```python
from build123d import *

# Parameters (mm, degrees)
SKETCH1_W           = 230
SKETCH1_H           = 25
BOSS_EXTRUDE1_DEPTH = 150
SKETCH2_W           = 210
SKETCH2_H           = 130
CUT_EXTRUDE1_DEPTH  = 20
SKETCH4_W           = 6.527967864
SKETCH4_H           = 110
BOSS_EXTRUDE3_DEPTH = 30
CUT_EXTRUDE2_REACH  = 7
SKETCH5_R           = 1.35
SKETCH5_R_2         = 1.5
SKETCH6_R           = 1.5
CUT_EXTRUDE3_DEPTH  = 6
CUT_EXTRUDE4_REACH  = 232
SKETCH7_R           = 3.25
CUT_EXTRUDE5_REACH  = 12
SKETCH8_R           = 3.25
SKETCH9_W           = 4.75
SKETCH9_H           = 80
BOSS_EXTRUDE4_DEPTH = 10
SKETCH10_R          = 2
CUT_EXTRUDE6_DEPTH  = 10
SKETCH11_R          = 2
CUT_EXTRUDE7_DEPTH  = 10
SKETCH12_W          = 3.25
SKETCH12_H          = 7.5
CUT_EXTRUDE8_DEPTH  = 8.5
SKETCH13_W          = 4.75
SKETCH13_H          = 1
CUT_EXTRUDE9_DEPTH  = 10


with BuildPart() as part:
    # Sketch1 → Boss-Extrude1 (new body)
    with BuildSketch(Plane.XY):
        with Locations((115, 12.5)):
            Rectangle(SKETCH1_W, SKETCH1_H)
    extrude(amount=BOSS_EXTRUDE1_DEPTH)

    # Sketch2 → Cut-Extrude1 (cut)
    with BuildSketch(Plane(origin=(0, 25, 0), x_dir=(1, 0, 0), z_dir=(0, 1, 0))):
        with Locations((115, -75)):
            Rectangle(SKETCH2_W, SKETCH2_H)
    extrude(amount=-CUT_EXTRUDE1_DEPTH, mode=Mode.SUBTRACT)

    # Sketch4 → Boss-Extrude3 (add)
    with BuildSketch(Plane(origin=(0, 5, 0), x_dir=(1, 0, 0), z_dir=(0, 1, 0))):
        with Locations((56.736016068, -85)):
            Rectangle(SKETCH4_W, SKETCH4_H)
    extrude(amount=BOSS_EXTRUDE3_DEPTH)

    # Sketch5 → Cut-Extrude2 (cut, up to next)
    with BuildSketch(Plane(origin=(0, 5, 0), x_dir=(1, 0, 0), z_dir=(0, 1, 0)), mode=Mode.PRIVATE) as cut_extrude2_sk1:
        with Locations((67, -65)):
            Circle(SKETCH5_R)
    cut_extrude2_tool1 = extrude(cut_extrude2_sk1.sketch, amount=-CUT_EXTRUDE2_REACH, mode=Mode.PRIVATE) & part.part
    add(cut_extrude2_tool1.solids().sort_by_distance((67, 5, 65))[0], mode=Mode.SUBTRACT)
    # Sketch5 → Cut-Extrude2 (cut, up to next)
    with BuildSketch(Plane(origin=(0, 5, 0), x_dir=(1, 0, 0), z_dir=(0, 1, 0)), mode=Mode.PRIVATE) as cut_extrude2_sk2:
        with Locations((67, -114)):
            Circle(SKETCH5_R)
    cut_extrude2_tool2 = extrude(cut_extrude2_sk2.sketch, amount=-CUT_EXTRUDE2_REACH, mode=Mode.PRIVATE) & part.part
    add(cut_extrude2_tool2.solids().sort_by_distance((67, 5, 114))[0], mode=Mode.SUBTRACT)
    # Sketch5 → Cut-Extrude2 (cut, up to next)
    with BuildSketch(Plane(origin=(0, 5, 0), x_dir=(1, 0, 0), z_dir=(0, 1, 0)), mode=Mode.PRIVATE) as cut_extrude2_sk3:
        with Locations((125, -65)):
            Circle(SKETCH5_R_2)
    cut_extrude2_tool3 = extrude(cut_extrude2_sk3.sketch, amount=-CUT_EXTRUDE2_REACH, mode=Mode.PRIVATE) & part.part
    add(cut_extrude2_tool3.solids().sort_by_distance((125, 5, 65))[0], mode=Mode.SUBTRACT)
    # Sketch5 → Cut-Extrude2 (cut, up to next)
    with BuildSketch(Plane(origin=(0, 5, 0), x_dir=(1, 0, 0), z_dir=(0, 1, 0)), mode=Mode.PRIVATE) as cut_extrude2_sk4:
        with Locations((125, -114)):
            Circle(SKETCH5_R)
    cut_extrude2_tool4 = extrude(cut_extrude2_sk4.sketch, amount=-CUT_EXTRUDE2_REACH, mode=Mode.PRIVATE) & part.part
    add(cut_extrude2_tool4.solids().sort_by_distance((125, 5, 114))[0], mode=Mode.SUBTRACT)

    # Sketch6 → Cut-Extrude3 (cut, through all)
    with BuildSketch(Plane(origin=(0, 5, 0), x_dir=(1, 0, 0), z_dir=(0, 1, 0))):
        with Locations((132.15, -20.25)):
            Circle(SKETCH6_R)
        with Locations((169.85, -20.25)):
            Circle(SKETCH6_R)
        with Locations((169.85, -57.75)):
            Circle(SKETCH6_R)
        with Locations((132.15, -57.75)):
            Circle(SKETCH6_R)
        with Locations((178, -51.25)):
            Circle(SKETCH6_R)
        with Locations((215.7, -51.25)):
            Circle(SKETCH6_R)
        with Locations((215.7, -88.75)):
            Circle(SKETCH6_R)
        with Locations((178, -88.75)):
            Circle(SKETCH6_R)
        with Locations((156.15, -97.25)):
            Circle(SKETCH6_R)
        with Locations((193.85, -97.25)):
            Circle(SKETCH6_R)
        with Locations((193.85, -134.75)):
            Circle(SKETCH6_R)
        with Locations((156.15, -134.75)):
            Circle(SKETCH6_R)
    extrude(amount=-CUT_EXTRUDE3_DEPTH, mode=Mode.SUBTRACT)

    # Sketch7 → Cut-Extrude4 (cut, up to next)
    with BuildSketch(Plane.ZY, mode=Mode.PRIVATE) as cut_extrude4_sk1:
        with Locations((37.5, 12.5)):
            Circle(SKETCH7_R)
    cut_extrude4_tool1 = extrude(cut_extrude4_sk1.sketch, amount=-CUT_EXTRUDE4_REACH, mode=Mode.PRIVATE) & part.part
    add(cut_extrude4_tool1.solids().sort_by_distance((0, 12.5, 37.5))[0], mode=Mode.SUBTRACT)
    # Sketch7 → Cut-Extrude4 (cut, up to next)
    with BuildSketch(Plane.ZY, mode=Mode.PRIVATE) as cut_extrude4_sk2:
        with Locations((112.5, 12.5)):
            Circle(SKETCH7_R)
    cut_extrude4_tool2 = extrude(cut_extrude4_sk2.sketch, amount=-CUT_EXTRUDE4_REACH, mode=Mode.PRIVATE) & part.part
    add(cut_extrude4_tool2.solids().sort_by_distance((0, 12.5, 112.5))[0], mode=Mode.SUBTRACT)

    # Sketch8 → Cut-Extrude5 (cut, up to next)
    with BuildSketch(Plane.ZY.offset(-220), mode=Mode.PRIVATE) as cut_extrude5_sk1:
        with Locations((112.5, 12.5)):
            Circle(SKETCH8_R)
    cut_extrude5_tool1 = extrude(cut_extrude5_sk1.sketch, amount=-CUT_EXTRUDE5_REACH, mode=Mode.PRIVATE) & part.part
    add(cut_extrude5_tool1.solids().sort_by_distance((220, 12.5, 112.5))[0], mode=Mode.SUBTRACT)
    # Sketch8 → Cut-Extrude5 (cut, up to next)
    with BuildSketch(Plane.ZY.offset(-220), mode=Mode.PRIVATE) as cut_extrude5_sk2:
        with Locations((37.5, 12.5)):
            Circle(SKETCH8_R)
    cut_extrude5_tool2 = extrude(cut_extrude5_sk2.sketch, amount=-CUT_EXTRUDE5_REACH, mode=Mode.PRIVATE) & part.part
    add(cut_extrude5_tool2.solids().sort_by_distance((220, 12.5, 37.5))[0], mode=Mode.SUBTRACT)

    # Sketch9 → Boss-Extrude4 (add)
    with BuildSketch(Plane(origin=(0, 25, 0), x_dir=(1, 0, 0), z_dir=(0, 1, 0))):
        with Locations((5, -75)):
            Rectangle(SKETCH9_W, SKETCH9_H)
        with Locations((225, -75)):
            Rectangle(SKETCH9_W, SKETCH9_H)
    extrude(amount=BOSS_EXTRUDE4_DEPTH)

    # Sketch10 → Cut-Extrude6 (cut)
    with BuildSketch(Plane.ZY.offset(-2.625)):
        with Locations((55, 30)):
            Circle(SKETCH10_R)
        with Locations((75, 30)):
            Circle(SKETCH10_R)
        with Locations((95, 30)):
            Circle(SKETCH10_R)
    extrude(amount=-CUT_EXTRUDE6_DEPTH, mode=Mode.SUBTRACT)

    # Sketch11 → Cut-Extrude7 (cut)
    with BuildSketch(Plane.ZY.offset(-222.625)):
        with Locations((95, 30)):
            Circle(SKETCH11_R)
        with Locations((75, 30)):
            Circle(SKETCH11_R)
        with Locations((55, 30)):
            Circle(SKETCH11_R)
    extrude(amount=-CUT_EXTRUDE7_DEPTH, mode=Mode.SUBTRACT)

    # Sketch12 → Cut-Extrude8 (cut)
    with BuildSketch(Plane(origin=(0, 35, 0), x_dir=(1, 0, 0), z_dir=(0, 1, 0))):
        with Locations((5, -75)):
            Rectangle(SKETCH12_W, SKETCH12_H)
        with Locations((5, -95)):
            Rectangle(SKETCH12_W, SKETCH12_H)
        with Locations((5, -55)):
            Rectangle(SKETCH12_W, SKETCH12_H)
        with Locations((225, -95)):
            Rectangle(SKETCH12_W, SKETCH12_H)
        with Locations((225, -75)):
            Rectangle(SKETCH12_W, SKETCH12_H)
        with Locations((225, -55)):
            Rectangle(SKETCH12_W, SKETCH12_H)
    extrude(amount=-CUT_EXTRUDE8_DEPTH, mode=Mode.SUBTRACT)

    # Sketch13 → Cut-Extrude9 (cut)
    with BuildSketch(Plane(origin=(0, 35, 0), x_dir=(1, 0, 0), z_dir=(0, 1, 0))):
        with Locations((225, -35.5)):
            Rectangle(SKETCH13_W, SKETCH13_H)
        with Locations((225, -114.5)):
            Rectangle(SKETCH13_W, SKETCH13_H)
        with Locations((5, -35.5)):
            Rectangle(SKETCH13_W, SKETCH13_H)
        with Locations((5, -114.5)):
            Rectangle(SKETCH13_W, SKETCH13_H)
    extrude(amount=-CUT_EXTRUDE9_DEPTH, mode=Mode.SUBTRACT)


solid = part.part
```
Input: part model. Units: mm. Frame: model coordinates. A direction names the side the tool comes from. Coordinates: 2 decimals unless noted, no trailing zeros. Loops run counter-clockwise (first coordinate to the right, second up) from the corner with the lowest first, then second, coordinate; pieces in that order, holes last. Notation, with made-up numbers: (79, 81) -> (138, 81) arc R30 ccw to (138, 113) -> close; hole circle Ø1 at (40, -12). An arc over 180 degrees is marked (long way). Use a Markdown table: item, result.
1) Material intervals for line 1 along Z through (x, y) = (132.15, 2); line 2 along X through (y, z) = (9.5, 80); line 3 along X through (y, z) = (1.55, 57.75), sorted ascending. Write a range as from..to.
Results found:
| item | result |
|---|---|
| line 1 | z = 0..18.75, 21.75..56.25, 59.25..150 |
| line 2 | x = 0..10, 53.47..60, 220..230 |
| line 3 | x = 0..130.65, 133.65..168.35, 171.35..230 |
2) Cut plane A-A (x = 174). Return the cut outline in (y, z).
Results found:
| item | result |
|---|---|
| outline | (0, 0) -> (25, 0) -> (25, 10) -> (5, 10) -> (5, 140) -> (25, 140) -> (25, 150) -> (0, 150) -> close |
3) Pull-direction query (Y, two-part tool) for faces 5 (the flat face through (57, 20, 30)), 6 (the flat face through (57, 35, 84)), 7 (the cylindrical face through (224.93, 12.643, 109.253)); classes: released by +Y, released by -Y, zero draft, split by the parting line, or undercut.
Results found:
| item | result |
|---|---|
| face 5 | zero draft |
| face 6 | released by +Y |
| face 7 | undercut |
4) Contact query for flat-ended pins moving along their axis: pin 1 (2 mm diameter, centred on x = 145, z = 21, fed in from +Y); pin 2 (2 mm diameter, centred on x = 67, z = 114, fed in from -Y); pin 3 (3.5 mm diameter, centred on y = 30, z = 75, fed in from -X); pin 4 (4.5 mm diameter, centred on y = 30, z = 95, fed in from -X) (3 decimals). Output: stop coordinate, or through.
Results found:
| item | result |
|---|---|
| pin 1 | stops at y = 5 |
| pin 2 | passes through |
| pin 3 | stops at x = 53.47 |
| pin 4 | stops at x = 2.625 |
5) Access query for faces 1 (the cylindrical face through (224.93, 13.48, 40.6)), 2 (the flat face through (225, 30, 36)), 3 (the flat face through (5, 30, 114)), 4 (the flat face through (226.625, 33, 75)). Directions: +Z, -Z, +X, -X, +Y, -Y. A direction counts if a zero-diameter tool reaches every point of the face in a straight line with its end or side. Return the directions, or none.
Results found:
| item | result |
|---|---|
| face 1 | +X |
| face 2 | -Z, +X, +Y |
| face 3 | +Z, -X, +Y |
| face 4 | +Y |
